Part print with two shaded views. Sizes in mm from the minimum x, y, z corner. A direction names the side the tool comes from. Coordinates: 2 decimals unless noted, no trailing zeros. Write each loop counter-clockwise with the first axis right and the second up, starting at its lowest first coordinate (ties: lowest second). Pieces come first, ordered by that corner, then holes. Notation, with made-up numbers: (31.25, 8) - (53.25, 8) arc R18 ccw to (53.25, 12) - close; hole circle Ø4 at (-3, -15). An arc over 180 degrees is marked (long way). Answer in a Markdown table with one row per item. Add a question column.
Q1. Band-saw the part on C-C (x = 18.5). List the corners of the cut face in (y, z), and give its area (3 significant figures).
Q2. Band-saw the part on B-B (x = 8). List the corners of the cut face in (y, z).
Q3. Band-saw the part on A-A (y = 6). List the corners of the cut face in (x, z) (3 decimals), and give its area (3 significant figures).
Q4. Drill centre line: line 1 along Z through (x, y) = (5, 1.5). Where is it in solid material? Low to high. Write a range as from..to.
Q5. Pin check, flat tips, straight feed: pin 1 (4 mm diameter, centred on y = 4.5, z = 134, fed in from -X) (3 decimals); pin 2 (1.5 mm diameter, centred on x = 9.5, y = 1, fed in from +Z); pin 3 (1 mm diameter, centred on x = 11, y = 9, fed in from -Z). Stop position of each tip, or through.
Q6. 3-axis set-ups, long thin cutter, end or side, ignore diameter. For the marked faces 1, 2 and 3: which of +Z, -Z, +X, -X, +Y, -Y reach the whole face in a straight line?
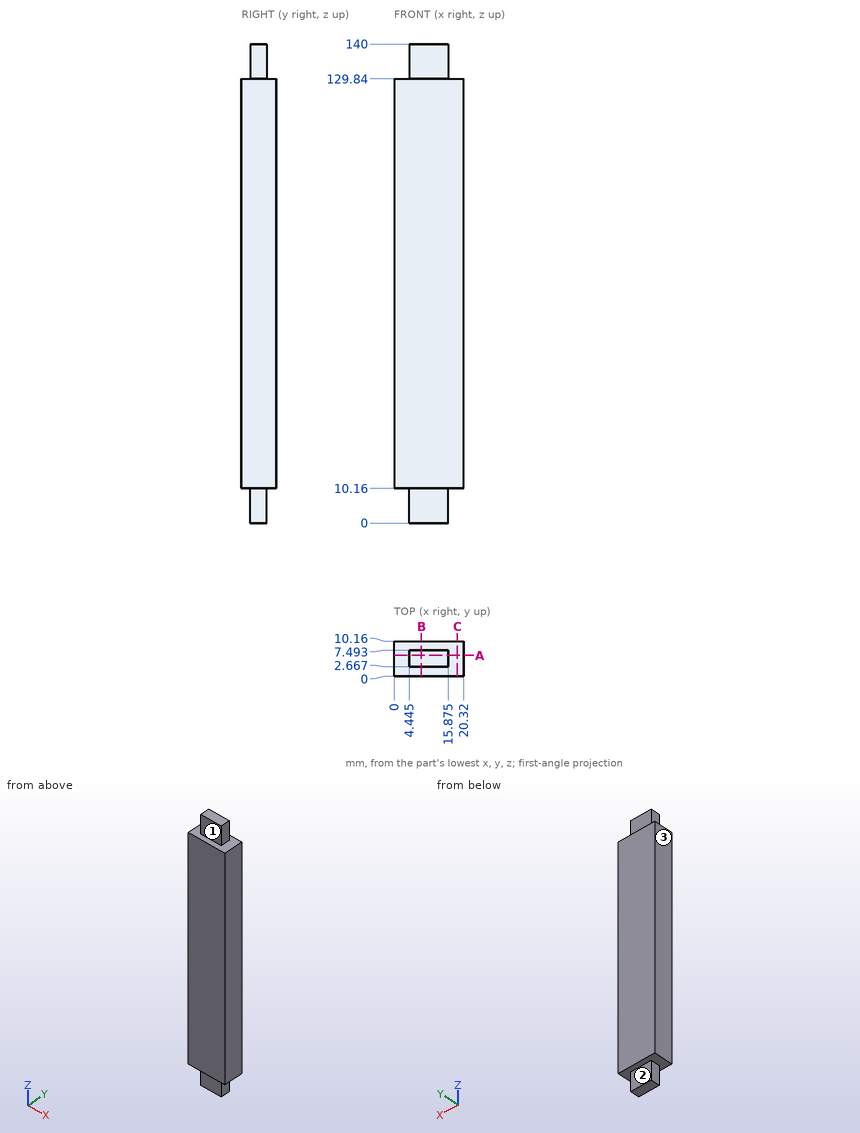
Checked values:
| question | item | result |
|---|---|---|
| 1 | outline | (0, 10.16) - (10.16, 10.16) - (10.16, 129.84) - (0, 129.84) - close |
| 1 | area | 1,220 mm² |
| 2 | outline | (0, 10.16) - (2.67, 10.16) - (2.67, 0) - (7.49, 0) - (7.49, 10.16) - (10.16, 10.16) - (10.16, 129.84) - (7.49, 129.84) - (7.49, 140) - (2.67, 140) - (2.67, 129.84) - (0, 129.84) - close |
| 3 | outline | (0, 10.16) - (4.445, 10.16) - (4.445, 0) - (15.875, 0) - (15.875, 10.16) - (20.32, 10.16) - (20.32, 129.84) - (15.875, 129.84) - (15.875, 140) - (4.445, 140) - (4.445, 129.84) - (0, 129.84) - close |
| 3 | area | 2,660 mm² |
| 4 | line 1 | z = 10.16..129.84 |
| 5 | pin 1 | stops at x = 4.445 |
| 5 | pin 2 | stops at z = 129.84 |
| 5 | pin 3 | stops at z = 10.16 |
| 6 | face 1 | +Z, +X, -X, -Y |
| 6 | face 2 | -Z, +X, -X, +Y |
| 6 | face 3 | +Z, -Z, -X, +Y, -Y |
